from build123d import *

# Parameters (mm, degrees)
EXTRUDE_1_DEPTH          = 10
CUT_EXTRUDE_1_DEPTH      = 19
SKETCH_9_R               = 3
EXTRUDE_2_DEPTH          = 2
SKETCH_11_R              = 2.5
EXTRUDE_4_DEPTH          = 24
SKETCH_12_W              = 3
SKETCH_12_H              = 4.5
CUT_EXTRUDE_2_DEPTH      = 4
CUT_EXTRUDE_2_DEPTH_BACK = 16
CUT_EXTRUDE_3_REACH      = 61
SKETCH_13_R              = 1.5
SKETCH_15_R              = 1.5
CUT_EXTRUDE_4_DEPTH      = 5


with BuildPart() as part:
    # 草图1 → 凸台-拉伸1 (new body)
    with BuildSketch(Plane.XY):
        Polygon((-15, -25.086741331), (-15, 7.913258669), (3, 7.913258669), (3, -25.086741331), (0, -25.086741331), (0, 2.913258669), (-12, 2.913258669), (-12, -25.086741331), align=None)
    extrude(amount=EXTRUDE_1_DEPTH)

    # 草图2 → 切除-拉伸1 (cut, through all)
    with BuildSketch(Plane(origin=(3, 0, 0), x_dir=(0, 0, -1), z_dir=(1, 0, 0))):
        with BuildLine():
            Line((-6.5, -20.086741331), (-6.5, -25.086741331))
            Line((-6.5, -25.086741331), (-3.5, -25.086741331))
            Line((-3.5, -25.086741331), (-3.5, -20.086741331))
            ThreePointArc((-3.5, -20.086741331), (-5, -18.586741331), (-6.5, -20.086741331))
        make_face()
    extrude(amount=-CUT_EXTRUDE_1_DEPTH, mode=Mode.SUBTRACT)

    # 草图9 → 凸台-拉伸2 (add)
    with BuildSketch(Plane(origin=(0, 7.913258669, 0), x_dir=(1, 0, 0), z_dir=(0, 1, 0))):
        with Locations((-6, -5)):
            Circle(SKETCH_9_R)
    extrude(amount=EXTRUDE_2_DEPTH)

    # 草图11 → 凸台-拉伸4 (add)
    with BuildSketch(Plane(origin=(0, 9.913258669, 0), x_dir=(1, 0, 0), z_dir=(0, 1, 0))):
        with Locations((-6, -5)):
            Circle(SKETCH_11_R)
    extrude(amount=EXTRUDE_4_DEPTH)

    # 草图12 → 切除-拉伸2 (cut, two sides)
    with BuildSketch(Plane(origin=(0, 0, 0), x_dir=(0, 0, -1), z_dir=(1, 0, 0))) as cut_extrude_2_sk:
        with Locations((-5, 28.163258669)):
            Rectangle(SKETCH_12_W, SKETCH_12_H)
    extrude(amount=CUT_EXTRUDE_2_DEPTH, mode=Mode.SUBTRACT)
    extrude(cut_extrude_2_sk.sketch, amount=-CUT_EXTRUDE_2_DEPTH_BACK, mode=Mode.SUBTRACT)

    # 草图13 → 切除-拉伸3 (cut, up to next)
    with BuildSketch(Plane(origin=(0, 33.913258669, 0), x_dir=(-1, 0, 0), z_dir=(0, 1, 0)), mode=Mode.PRIVATE) as cut_extrude_3_sk1:
        with Locations((6, 5)):
            Circle(SKETCH_13_R)
    cut_extrude_3_tool1 = extrude(cut_extrude_3_sk1.sketch, amount=-CUT_EXTRUDE_3_REACH, mode=Mode.PRIVATE) & part.part
    add(cut_extrude_3_tool1.solids().sort_by_distance((-6, 33.913259, 5))[0], mode=Mode.SUBTRACT)

    # 草图15 → 切除-拉伸4 (cut, symmetric)
    with BuildSketch(Plane.XY.offset(5)):
        with Locations((-6, 28.163258669)):
            Circle(SKETCH_15_R)
    extrude(amount=CUT_EXTRUDE_4_DEPTH, both=True, mode=Mode.SUBTRACT)


solid = part.part
Geometry check sheet. Reference: the model listing, model coordinates, mm. A direction names the side the tool comes from. Coordinates: 2 decimals unless noted, no trailing zeros. Order: outer loops, then holes, each group sorted by start corner. A loop starts at its lowest first (then second) coordinate and runs counter-clockwise, first axis right, second up. Notation, with made-up numbers: (-7, 63.25) -> (32, 63.25) arc R15 ccw to (32, 74.25) -> close; hole circle Ø5 at (88.5, -32.5). An arc over 180 degrees is marked (long way). Use a Markdown table: item, result. Add a question column.
1. Set-up check for faces 5 (the face through (2, -23, 3.5)), 6 (the face through (-12, -11, 5)), 7 (the face through (-8.5, 21.7, 4.9)): record each of +Z, -Z, +X, -X, +Y, -Y from which the full face is reachable in a straight line by a thin tool's end or side.
2. Mould release check, pull along Y, two halves, no side actions. Record for faces 1 (the face through (-6.1, 7.913, 1.6)), 2 (the face through (-7.106, 29.177, 3.118)), 3 (the face through (-13.479, -18.587, 4.967)), 4 (the face through (-4.8, 32.2, 4.1)): pulls with the +Y half, pulls with the -Y half, needs draft (parallel to the pull), parting line crosses it, or undercut.
3. Go/stop test with flat-tipped pins: pin 1 Ø1.2 at (x, z) = (-4.5, 4.5) entering from -Y; pin 2 Ø3 at (y, z) = (14, 6) entering from -X; pin 3 Ø1.8 at (x, z) = (-5.5, 5) entering from +Y. Record where each tip stops, or that it passes through.
4. Cross-section at A-A (x = 0.5). Enter the section's corners in (y, z).
5. Material ranges on L1, parallel to X at y = 32.7, z = 5; L2, parallel to X at y = 0.5, z = 4.75; L3, parallel to Z at x = -6, y = 32, recorded low to high.
6. Cross-section at D-D (x = -5.25). Enter the section's corners in (y, z).
7. Cross-section at B-B (y = -5.5). Enter the section's corners in (x, z).
8. Cross-section at C-C (z = 5). Enter the section's corners in (x, y), and give its area (3 significant figures).
Filled sheet:
| question | item | result |
|---|---|---|
| 1 | face 5 | +X, -X, -Y |
| 1 | face 6 | +Z, -Z, -Y |
| 1 | face 7 | +Y |
| 2 | face 1 | pulls with the +Y half |
| 2 | face 2 | undercut |
| 2 | face 3 | pulls with the -Y half |
| 2 | face 4 | needs draft |
| 3 | pin 1 | y = 2.91 |
| 3 | pin 2 | x = -8.5 |
| 3 | pin 3 | y = 25.91 |
| 4 | outline | (-25.09, 0) -> (7.91, 0) -> (7.91, 10) -> (-25.09, 10) -> (-25.09, 6.5) -> (-20.09, 6.5) arc R1.5 cw to (-20.09, 3.5) -> (-25.09, 3.5) -> close |
| 5 | L1 | -8.5 to -7.5, -4.5 to -3.5 |
| 5 | L2 | -15 to -12, 0 to 3 |
| 5 | L3 | 2.5 to 3.5, 6.5 to 7.5 |
| 6 | outline | (2.91, 0) -> (7.91, 0) -> (7.91, 2.1) -> (9.91, 2.1) -> (9.91, 2.62) -> (26.86, 2.62) -> (26.86, 3.5) -> (25.91, 3.5) -> (25.91, 6.5) -> (26.86, 6.5) -> (26.86, 7.38) -> (9.91, 7.38) -> (9.91, 7.9) -> (7.91, 7.9) -> (7.91, 10) -> (2.91, 10) -> close; (29.46, 2.62) -> (33.91, 2.62) -> (33.91, 3.7) -> (30.41, 3.7) -> (30.41, 3.5) -> (29.46, 3.5) -> close; (29.46, 6.5) -> (30.41, 6.5) -> (30.41, 6.3) -> (33.91, 6.3) -> (33.91, 7.38) -> (29.46, 7.38) -> close |
| 7 | outline | (-15, 0) -> (-12, 0) -> (-12, 10) -> (-15, 10) -> close; (0, 0) -> (3, 0) -> (3, 10) -> (0, 10) -> close |
| 8 | outline | (-15, -18.59) -> (-12, -18.59) -> (-12, 2.91) -> (0, 2.91) -> (0, -18.59) -> (3, -18.59) -> (3, 7.91) -> (-3, 7.91) -> (-3, 9.91) -> (-3.5, 9.91) -> (-3.5, 25.91) -> (-8.5, 25.91) -> (-8.5, 9.91) -> (-9, 9.91) -> (-9, 7.91) -> (-15, 7.91) -> close; (-8.5, 30.41) -> (-7.5, 30.41) -> (-7.5, 33.91) -> (-8.5, 33.91) -> close; (-4.5, 30.41) -> (-3.5, 30.41) -> (-3.5, 33.91) -> (-4.5, 33.91) -> close |
| 8 | area | 318 mm2 |
